Geometry check sheet. Reference: drawing and pictorial views, mm from the part's lowest x, y, z. A direction names the side the tool comes from. Coordinates: 2 decimals unless noted, no trailing zeros. Loops run counter-clockwise (first coordinate to the right, second up) from the corner with the lowest first, then second, coordinate; pieces in that order, holes last. Notation, with made-up numbers: (11, 47.25) - (45, 47.25) arc R17 ccw to (45, 52.25) - close; hole circle Ø9 at (-14, 20.25). An arc over 180 degrees is marked (long way). One line per item, written item: value.
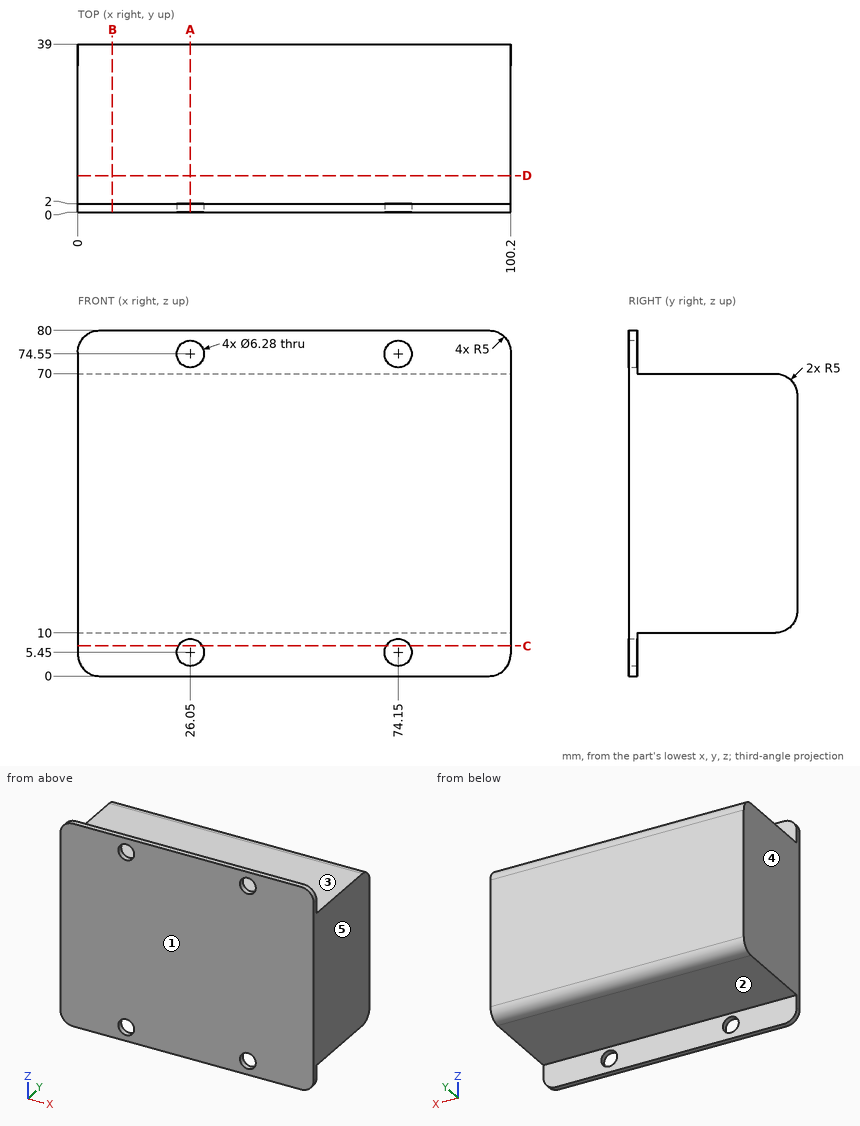
(1) Access from +Z, -Z, +X, -X, +Y, -Y to the whole of each face (thin tool, end or side, straight path). Record for the marked faces 1 and 2.
Reply:
face 1: +Z, -Z, +X, -X, -Y
face 2: -Z, +X, -X, +Y
(2) Cross-section at D-D on y = 8.5. Record the cut outline in (x, z).
Reply:
outline: (0, 10) - (100.2, 10) - (100.2, 70) - (0, 70) - close
(3) Go/stop test with flat-tipped pins: pin 1 Ø1 at (x, y) = (22, 7) entering from +Z; pin 2 Ø8 at (x, z) = (51, 77) entering from +Y. Record where each tip stops, or that it passes through.
Reply:
pin 1: z = 70
pin 2: y = 2
(4) Cross-section at A-A on x = 26.05. Record the cut outline in (y, z), and give its area (3 significant figures).
Reply:
outline: (0, 0) - (2, 0) - (2, 2.31) - (0, 2.31) - close; (0, 8.59) - (2, 8.59) - (2, 10) - (34, 10) arc R5 ccw to (39, 15) - (39, 65) arc R5 ccw to (34, 70) - (2, 70) - (2, 71.41) - (0, 71.41) - close; (0, 77.69) - (2, 77.69) - (2, 80) - (0, 80) - close
area: 2,340 mm2
(5) Cross-section at B-B on x = 8. Record the cut outline in (y, z).
Reply:
outline: (0, 0) - (2, 0) - (2, 10) - (34, 10) arc R5 ccw to (39, 15) - (39, 65) arc R5 ccw to (34, 70) - (2, 70) - (2, 80) - (0, 80) - close
(6) Material ranges on probe 1 along X at (y, z) = (1.15, 74.55); probe 2 along Z at (x, y) = (74.15, 0.6); probe 3 along Z at (x, y) = (6.5, 31), recorded low to high. Write a range as from..to.
Reply:
probe 1: 0..22.91, 29.19..71.01, 77.29..100.2
probe 2: 0..2.31, 8.59..71.41, 77.69..80
probe 3: 10..70
(7) Release check for a two-part mould opening along X. For the marked faces 3, 4 and 5 record: pulls with the +X half, pulls with the -X half, needs draft (parallel to the pull), parting line crosses it, or undercut.
Reply:
face 3: needs draft
face 4: pulls with the -X half
face 5: pulls with the +X half
(8) Cross-section at C-C on z = 7. Record the cut outline in (x, y), and give its area (3 significant figures).
Reply:
outline: (0, 0) - (23.32, 0) - (23.32, 2) - (0, 2) - close; (28.78, 0) - (71.42, 0) - (71.42, 2) - (28.78, 2) - close; (76.88, 0) - (100.2, 0) - (100.2, 2) - (76.88, 2) - close
area: 179 mm2
